Input: dimensioned drawing with shaded views. Units: mm. Origin: part minimum x, y, z. Give positions to 0.01 mm unless a question says otherwise; leave off trailing zeros. Order: outer loops, then holes, each group sorted by start corner. A loop starts at its lowest first (then second) coordinate and runs counter-clockwise, first axis right, second up. Notation, with made-up numbers: (-11, -28) -> (4, -28) arc R32 ccw to (4, 9) -> close; hole circle Ø4 at (15.5, -2.75). An arc over 180 degrees is marked (long way). Use CSV: the item, a comma, the result in double quotes.
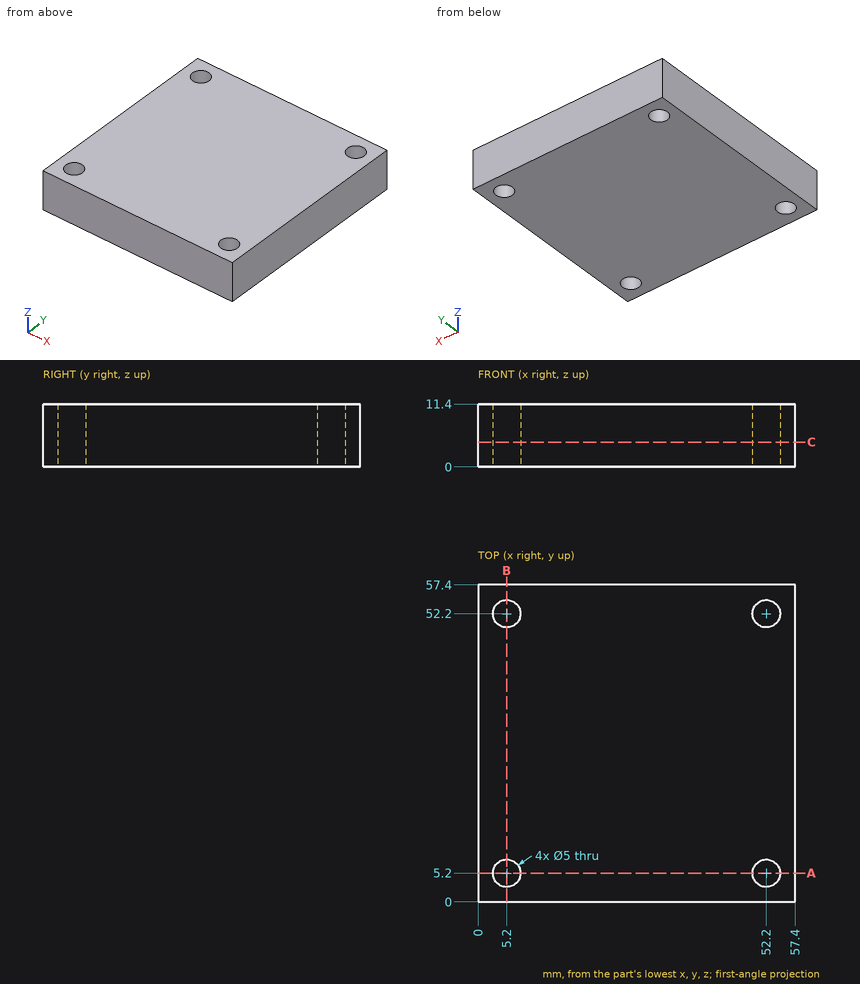
1. Section query C-C on z = 4.5. Return loops of the section in (x, y).
Answer below:
outline,"(0, 0) -> (57.4, 0) -> (57.4, 57.4) -> (0, 57.4) -> close; hole circle Ø5 at (5.2, 5.2); hole circle Ø5 at (5.2, 52.2); hole circle Ø5 at (52.2, 5.2); hole circle Ø5 at (52.2, 52.2)"
2. Ray query, line 1 along X through (y, z) = (52, 9.25); line 2 along Y through (x, z) = (5.2, 8); line 3 along X through (y, z) = (51, 6). Return the intervals inside material, ascending.
Answer below:
line 1,"x = 0 to 2.71, 7.69 to 49.71, 54.69 to 57.4"
line 2,"y = 0 to 2.7, 7.7 to 49.7, 54.7 to 57.4"
line 3,"x = 0 to 3.01, 7.39 to 50.01, 54.39 to 57.4"
3. Section query A-A on y = 5.2. Return loops of the section in (x, z), plus the area to 3 significant figures.
Answer below:
outline,"(0, 0) -> (2.7, 0) -> (2.7, 11.4) -> (0, 11.4) -> close; (7.7, 0) -> (49.7, 0) -> (49.7, 11.4) -> (7.7, 11.4) -> close; (54.7, 0) -> (57.4, 0) -> (57.4, 11.4) -> (54.7, 11.4) -> close"
area,"540 mm²"
